from build123d import *

# Parameters (mm, degrees)
F1_DEPTH = 63.5
F0_W     = 25.4
F0_H     = 19.05
F2_DEPTH = 25.4
F3_DEPTH = 7.9375
F5_R     = 6.35
F6_R     = 20.6375
F7_DEPTH = 28.575


with BuildPart() as f1:
    # F0 (on Front) → F1 (new body, symmetric)
    with BuildSketch(Plane.XZ):
        Polygon((22.225, 9.525), (-41.275, 9.525), (-41.275, -9.525), (41.275, -9.525), (41.275, 9.525), align=None)
    extrude(amount=F1_DEPTH, both=True)

    # F0 (on Front) → F2 (join, symmetric)
    with BuildSketch(Plane.XZ):
        with BuildLine():
            Line((22.225, 26.9875), (22.225, 9.525))
            Line((22.225, 9.525), (41.275, 9.525))
            Line((41.275, 9.525), (41.275, 26.9875))
            ThreePointArc((41.275, 26.9875), (45.9246798487, 38.2128201513), (57.15, 42.8625))
            Line((57.15, 42.8625), (60.325, 42.8625))
            Line((60.325, 42.8625), (60.325, 61.9125))
            Line((60.325, 61.9125), (57.15, 61.9125))
            add(Edge.make_bspline(
                [(52.8412517036, 61.645692583), (54.2960084782, 61.7553557468), (55.7333080452, 61.8443643855), (57.15, 61.9125)],
                knots=[107.618064177, 107.618064177, 107.618064177, 107.618064177, 111.4985685166, 111.4985685166, 111.4985685166, 111.4985685166], degree=3))
            ThreePointArc((52.8412517036, 61.645692583), (30.9752157673, 50.1097035147), (22.225, 26.9875))
        make_face()
        with Locations((73.025, 52.3875)):
            Rectangle(F0_W, F0_H)
    extrude(amount=F2_DEPTH, both=True)

    # F0 (on Front) → F3 (join, symmetric)
    with BuildSketch(Plane.XZ):
        with BuildLine():
            add(Edge.make_bspline(
                [(-41.275, 9.525), (-41.275, 39.6773087956), (12.4964680785, 58.6044030066), (52.8412517036, 61.645692583)],
                knots=[0, 0, 0, 0, 107.618064177, 107.618064177, 107.618064177, 107.618064177], degree=3))
            Line((-41.275, 9.525), (22.225, 9.525))
            Line((22.225, 9.525), (22.225, 26.9875))
            ThreePointArc((22.225, 26.9875), (30.9752157673, 50.1097035147), (52.8412517036, 61.645692583))
        make_face()
    extrude(amount=F3_DEPTH, both=True)

    # F0 (on Front) → F4 (revolve)
    with BuildSketch(Plane.XZ):
        Polygon((85.725, 66.675), (85.725, 61.9125), (85.725, 42.8625), (85.725, 38.1), (111.125, 38.1), (111.125, 66.675), align=None)
    revolve(axis=Axis((85.725, 0, 52.3875), (0, 0, 1)))

    # F5
    f5_edges = [f1.edges().sort_by_distance(p)[0] for p in [
        (41.275, -63.5, 0),
        (-41.275, -63.5, 0),
        (41.275, 63.5, 0),
        (-41.275, 63.5, 0),
    ]]
    fillet(f5_edges, radius=F5_R)

    # F6 (on face) → F7 (cut, through all)
    with BuildSketch(Plane.XY.offset(66.675)):
        with Locations((85.725, 0)):
            Circle(F6_R)
    extrude(amount=-F7_DEPTH, mode=Mode.SUBTRACT)


solid = f1.part
Source: CAD feature listing. Evaluate the final solid. Frame: model axes, mm. A direction names the side the tool comes from. Coordinates: 2 decimals unless noted, no trailing zeros. Order: outer loops, then holes, each group sorted by start corner. A loop starts at its lowest first (then second) coordinate and runs counter-clockwise, first axis right, second up. Notation, with made-up numbers: M -10.5,30 L 40.5,30 A23 ccw 40.5,59 Z; hole C 38,67.5 d9. An arc over 180 degrees is marked long. Write each question's results on one line, items separated by ' | '. Start each with the question number.
1. Section B-B, the plane y = -33. Return the cut outline in (x, z) (3 decimals).
2. Material intervals for L1, parallel to Y at x = 27, z = 17; L2, parallel to X at y = -25, z = 22 (3 decimals); L3, parallel to X at y = 2, z = 63, sorted ascending.
3. Pin query (flat end, axial travel): pin 1 (1 mm diameter, centred on x = 42, y = -27, fed in from -Z); pin 2 (8.5 mm diameter, centred on y = 13, z = 16.5, fed in from -X) (3 decimals); pin 3 (2 mm diameter, centred on x = 69, z = 49.5, fed in from +Y); pin 4 (4 mm diameter, centred on x = -12, y = 33, fed in from +Z) (3 decimals). Return the tip coordinate at first contact, or that it passes through.
4. Reachability of faces 1 (the face through (-4, -7.938, 30)), 2 (the face through (60, -2, 61.912)), 3 (the face through (31.21, 16.55, 50.37)), 4 (the face through (46, 25.4, 42)) from +Z, -Z, +X, -X, +Y, -Y: full face, straight path, thin tool, end or side. Return the list, or none.
5. Section A-A, the plane x = 94. Return the cut outline in (y, z) (3 decimals).
Solution:
1) outline: M -41.275,-9.525 L 41.275,-9.525 L 41.275,9.525 L -41.275,9.525 Z
2) L1: -25.4 to 25.4 | L2: 22.225 to 41.275 | L3: 60.4 to 65.18, 106.27 to 111.05
3) pin 1: through | pin 2: x = 22.225 | pin 3: y = 25.4 | pin 4: z = 9.525
4) face 1: +Z, -X, -Y | face 2: +Z, -X | face 3: +Z, -X, +Y | face 4: +Z, +X, -X, +Y
5) outline: M -24.014,38.1 L -18.906,38.1 L -18.906,66.675 L -24.014,66.675 Z; M 18.906,38.1 L 24.014,38.1 L 24.014,66.675 L 18.906,66.675 Z
